Geometry check sheet. Reference: the model listing, model coordinates, mm. Face numbers are marked on the shaded views. A direction names the side the tool comes from. Give positions to 0.01 mm unless a question says otherwise; leave off trailing zeros. Order: outer loops, then holes, each group sorted by start corner. A loop starts at its lowest first (then second) coordinate and runs counter-clockwise, first axis right, second up. Notation, with made-up numbers: M 30,28.25 L 52,28.25 A16 cw 52,54.25 Z; hole C 16,76.5 d8. An arc over 180 degrees is marked long. Put each result on its own line as item: value. Start each with the question number.
Q1. Material ranges on L1, parallel to Y at x = 2.5, z = -10; L2, parallel to Z at x = 0, y = 3 (3 decimals); L3, parallel to X at y = 4.45, z = 0 (3 decimals), recorded low to high.
Q2. Section check C-C on y = 4. Record the cut outline in (x, z) (3 decimals), then the cut area to 3 significant figures.
Q3. Section check A-A on x = 15.5. Record the cut outline in (y, z), then the cut area to 3 significant figures.
Q4. Section check D-D on x = -11. Record the cut outline in (y, z), then the cut area to 3 significant figures.
Q5. Mould release check, pull along Z, two halves, no side actions. Record for the marked faces 4 and 5: +Z half, -Z half, draft (parallel to the pull), parting line (faces both ways), or undercut.
Q6. Access from +Z, -Z, +X, -X, +Y, -Y to the whole of each face (thin tool, end or side, straight path). Record for the marked faces 1, 2 and 3.
Q7. Go/stop test with flat-tipped pins: pin 1 (5 mm diameter, centred on x = 5.5, y = 3.5, fed in from +Z); pin 2 (1 mm diameter, centred on y = 3.5, z = -1, fed in from -X); pin 3 (1.5 mm diameter, centred on y = 3, z = 3, fed in from -X); pin 4 (7.5 mm diameter, centred on x = 0, z = 0, fed in from -Y). Record where each tip stops, or that it passes through.
Q8. Section check B-B on z = -15.5. Record the cut outline in (x, y), then the cut area to 3 significant figures.
```python
from build123d import *

# Parameters (mm, degrees)
BOSS_EXTRUDE1_DEPTH     = 3.556
CIRPATTERN1_COUNT       = 20
SKETCH2_W               = 10.342329408
SKETCH2_H               = 1.5875
SKETCH9_R               = 19.84375
SKETCH9_R_2             = 1.5
BOSS_EXTRUDE2_DEPTH     = 1.5875
SKETCH3_R               = 1.74625
CUT_EXTRUDE1_DEPTH      = 6.087499985
CUT_EXTRUDE1_DEPTH_BACK = 6.087499985
CIRPATTERN2_COUNT       = 4
SKETCH12_R              = 3.175
CUT_EXTRUDE2_DEPTH      = 3.175
SKETCH13_R              = 1.525
CUT_EXTRUDE4_DEPTH      = 7.99999997


with BuildPart() as part:
    # Sketch1 → Boss-Extrude1 (new body, symmetric)
    with BuildSketch(Plane(origin=(0, 0, 0), x_dir=(1, 0, 0), z_dir=(0, 1, 0))):
        with BuildLine():
            ThreePointArc((0.872060607, 8.659786465), (0.562967303, 8.148255135), (0, 7.947579308))
            ThreePointArc((0, 7.947579308), (-1.243275317, -7.849731418), (2.45593707, 7.55859709))
            ThreePointArc((2.45593707, 7.55859709), (1.982535589, 7.923417607), (1.846642263, 8.505427895))
            ThreePointArc((1.846642263, 8.505427895), (1.749626992, 8.862101959), (1.434119122, 9.054671776))
            ThreePointArc((1.434119122, 9.054671776), (1.074545959, 8.969024291), (0.872060607, 8.659786465))
        make_face()
    boss_extrude1 = extrude(amount=BOSS_EXTRUDE1_DEPTH, both=True)

    # CirPattern1: Boss-Extrude1 ×20 about axis
    cirpattern1_axis = Axis((0, 0, 0), (0, 1, 0))
    for i in range(1, CIRPATTERN1_COUNT):
        add(boss_extrude1.rotate(cirpattern1_axis, i * 360 / CIRPATTERN1_COUNT))

    # Sketch2 → Revolve3 (revolve)
    with BuildSketch(Plane(origin=(0, 0, 0), x_dir=(0, 0, -1), z_dir=(1, 0, 0))):
        with Locations((5.171164704, 4.293749985)):
            Rectangle(SKETCH2_W, SKETCH2_H)
    revolve3 = revolve(axis=Axis((0, 3.3, 0), (0, -1, 0)))

    # Mirror1: Revolve3 across plane
    add(revolve3.mirror(Plane.ZX))

    # Sketch9 → Boss-Extrude2 (add)
    with BuildSketch(Plane.XZ.offset(5.087499985)):
        Circle(SKETCH9_R)
        Circle(SKETCH9_R_2, mode=Mode.SUBTRACT)
    extrude(amount=-BOSS_EXTRUDE2_DEPTH)

    # Sketch3 → Cut-Extrude1 (cut, two sides)
    with BuildSketch(Plane(origin=(0, 0, 0), x_dir=(1, 0, 0), z_dir=(0, 1, 0))) as cut_extrude1_sk:
        with Locations((-15.5, 0)):
            Circle(SKETCH3_R)
        with Locations((0, 15.5)):
            Circle(SKETCH3_R)
        with Locations((15.5, 0)):
            Circle(SKETCH3_R)
        with Locations((0, -15.5)):
            Circle(SKETCH3_R)
    extrude(amount=CUT_EXTRUDE1_DEPTH, mode=Mode.SUBTRACT)
    extrude(cut_extrude1_sk.sketch, amount=-CUT_EXTRUDE1_DEPTH_BACK, mode=Mode.SUBTRACT)

    # Sketch6 → Cut-Revolve2 (revolve, cut)
    with BuildSketch(Plane.XY):
        Polygon((-11.8678, -3.499999985), (-15.5, -7.132199985), (-15.5, -3.499999985), align=None)
    cut_revolve2 = revolve(axis=Axis((-15.5, -5.087499985, 0), (0, 1, 0)), mode=Mode.SUBTRACT)

    # CirPattern2: Cut-Revolve2 ×4 about axis
    cirpattern2_axis = Axis((0, 0, 0), (0, 1, 0))
    for i in range(1, CIRPATTERN2_COUNT):
        add(cut_revolve2.rotate(cirpattern2_axis, i * 360 / CIRPATTERN2_COUNT), mode=Mode.SUBTRACT)

    # Sketch12 → Cut-Extrude2 (cut)
    with BuildSketch(Plane(origin=(0, 5.087499985, 0), x_dir=(1, 0, 0), z_dir=(0, 1, 0))):
        Circle(SKETCH12_R)
    extrude(amount=-CUT_EXTRUDE2_DEPTH, mode=Mode.SUBTRACT)

    # Sketch13 → Cut-Extrude4 (cut, through all)
    with BuildSketch(Plane(origin=(0, 1.912499985, 0), x_dir=(1, 0, 0), z_dir=(0, 1, 0))):
        Circle(SKETCH13_R)
    extrude(amount=-CUT_EXTRUDE4_DEPTH, mode=Mode.SUBTRACT)


solid = part.part
```
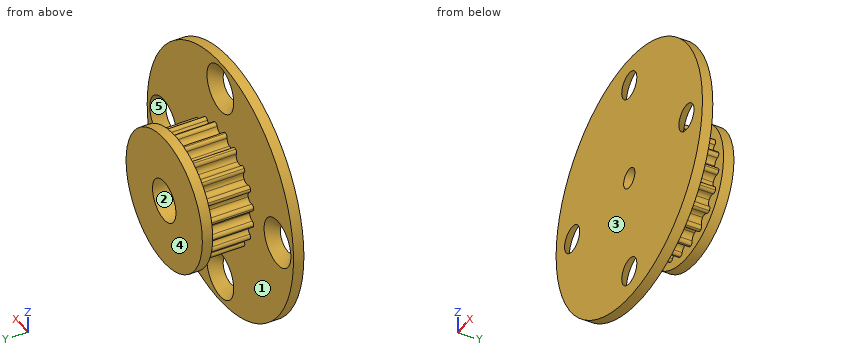
Results found:
1. L1: y = -5.09 to -3.5, 3.5 to 5.09
1. L2: z = -7.948 to -3.175, 3.175 to 7.948
1. L3: x = -10.342 to -3.175, 3.175 to 10.342
2. outline: C 0,0 d20.685; hole C 0,0 d6.35
2. area: 304 mm^2
3. outline: M -5.09,-12.39 L -3.5,-12.39 L -3.5,-3.63 L -5.09,-2.04 Z; M -5.09,2.04 L -3.5,3.63 L -3.5,12.39 L -5.09,12.39 Z
3. area: 30.3 mm^2
4. outline: M -5.09,-16.52 L -3.5,-16.52 L -3.5,16.52 L -5.09,16.52 Z
4. area: 52.4 mm^2
5. face 4: draft
5. face 5: undercut
6. face 1: none
6. face 2: +Y
6. face 3: +Z, -Z, +X, -X, -Y
7. pin 1: stops at z = 9.9
7. pin 2: stops at x = -10.33
7. pin 3: stops at x = -10.05
7. pin 4: stops at y = -5.09
8. outline: M -12.39,-5.09 L -2.04,-5.09 L -3.63,-3.5 L -12.39,-3.5 Z; M 2.04,-5.09 L 12.39,-5.09 L 12.39,-3.5 L 3.63,-3.5 Z
8. area: 30.3 mm^2
